Part model, mm, in its own coordinate system. A direction names the side the tool comes from. Give positions to 0.01 mm unless a question says otherwise; leave off trailing zeros. Loops run counter-clockwise (first coordinate to the right, second up) from the corner with the lowest first, then second, coordinate; pieces in that order, holes last. Notation, with made-up numbers: M 19.5,-18 L 36.5,-18 A22 ccw 36.5,4 Z; hole C 45.5,38.25 d11. An arc over 180 degrees is marked long. Answer in a Markdown table with one row per item.
from build123d import *

# Parameters (mm, degrees)
F0_W     = 600
F0_H     = 120
F1_DEPTH = 20
F2_W     = 20
F2_H     = 20
F3_DEPTH = 20
F4_W     = 559
F4_H     = 10
F5_DEPTH = 10


with BuildPart() as f1:
    # F0 (on Front) → F1 (new body)
    with BuildSketch(Plane.XZ):
        Rectangle(F0_W, F0_H)
    extrude(amount=F1_DEPTH)

    # F2 (on face) → F3 (cut, through all)
    with BuildSketch(Plane.XZ.offset(20)):
        with Locations((290, -30)):
            Rectangle(F2_W, F2_H)
        with Locations((290, 10)):
            Rectangle(F2_W, F2_H)
        with Locations((-290, 10)):
            Rectangle(F2_W, F2_H)
        with Locations((-290, -30)):
            Rectangle(F2_W, F2_H)
        with Locations((290, 50)):
            Rectangle(F2_W, F2_H)
        with Locations((-290, 50)):
            Rectangle(F2_W, F2_H)
    extrude(amount=-F3_DEPTH, mode=Mode.SUBTRACT)

    # F4 (on face) → F5 (cut)
    with BuildSketch(Plane(origin=(0, 0, 0), x_dir=(-1, 0, 0), z_dir=(0, 1, 0))):
        with Locations((0, -45)):
            Rectangle(F4_W, F4_H)
    extrude(amount=-F5_DEPTH, mode=Mode.SUBTRACT)


solid = f1.part
(1) Saw through at B-B (x = -120.5). Write the cut outline in (y, z).
Recorded:
| item | result |
|---|---|
| outline | M -20,-60 L 0,-60 L 0,-50 L -10,-50 L -10,-40 L 0,-40 L 0,60 L -20,60 Z |
(2) Drill centre lines: line 1 along X through (y, z) = (-4.75, -49); line 2 along Z through (x, y) = (-35.5, -3.5); line 3 along X through (y, z) = (-17.75, 46.5). Where is each one in solid material? Low to high.
Recorded:
| item | result |
|---|---|
| line 1 | x = -300 to -279.5, 279.5 to 300 |
| line 2 | z = -60 to -50, -40 to 60 |
| line 3 | x = -280 to 280 |
(3) Pin check, flat tips, straight feed: pin 1 Ø6 at (y, z) = (-8.5, 46.5) entering from -X; pin 2 Ø6 at (y, z) = (-8.5, 9.5) entering from +X; pin 3 Ø6 at (x, y) = (-286.5, -12) entering from +Z. Stop position of each tip, or through.
Recorded:
| item | result |
|---|---|
| pin 1 | stops at x = -280 |
| pin 2 | stops at x = 280 |
| pin 3 | stops at z = 40 |
(4) Which spindle directions (+Z, -Z, +X, -X, +Y, -Y) get a long thin tool onto all of the face, cutting with end or side? Do faces 1 (the face through (290, -10, 0)), 2 (the face through (-280, -10, 50)), 3 (the face through (4, -5, -50)). Say none if no direction does.
Recorded:
| item | result |
|---|---|
| face 1 | +X, +Y, -Y |
| face 2 | +Z, -X, +Y, -Y |
| face 3 | +Y |
(5) Pull direction Z, two halves, no side cores. Call faces 4 (the face through (300, -10, 30)), 5 (the face through (290, -10, -40)), 6 (the face through (-290, -10, 40)): +Z half, -Z half, draft (parallel to the pull), parting line (faces both ways), or undercut.
Recorded:
| item | result |
|---|---|
| face 4 | draft |
| face 5 | undercut |
| face 6 | +Z half |
(6) Saw through at A-A (y = -6.25). Write the cut outline in (x, z).
Recorded:
| item | result |
|---|---|
| outline | M -300,-60 L 300,-60 L 300,-40 L 280,-40 L 280,-20 L 300,-20 L 300,0 L 280,0 L 280,20 L 300,20 L 300,40 L 280,40 L 280,60 L -280,60 L -280,40 L -300,40 L -300,20 L -280,20 L -280,0 L -300,0 L -300,-20 L -280,-20 L -280,-40 L -300,-40 Z; hole M -279.5,-50 L 279.5,-50 L 279.5,-40 L -279.5,-40 Z |
